Verification items for the finished model (mm, model axes). Face numbers are marked on the shaded views. A direction names the side the tool comes from. Coordinates: 2 decimals unless noted, no trailing zeros. Order: outer loops, then holes, each group sorted by start corner. A loop starts at its lowest first (then second) coordinate and runs counter-clockwise, first axis right, second up. Notation, with made-up numbers: M 82,61.5 L 112,61.5 A17 cw 112,81.5 Z; hole C 85.5,-39 d6. An arc over 180 degrees is marked long. Use one line per item in the form item = value. Start each with the question number.
```python
from build123d import *

# Parameters (mm, degrees)
SKETCH1_W           = 3.5
SKETCH1_H           = 4
SKETCH2_R           = 2
BOSS_EXTRUDE1_DEPTH = 20
SKETCH3_R           = 2
BOSS_EXTRUDE2_DEPTH = 20
CUT_EXTRUDE1_DEPTH  = 2.4


with BuildPart() as part:
    # Sketch1 → Revolve1 (revolve)
    with BuildSketch(Plane.XZ, mode=Mode.PRIVATE) as revolve1_sk:
        with Locations((1.75, 2)):
            Rectangle(SKETCH1_W, SKETCH1_H)
    revolve(revolve1_sk.sketch.rotate(Axis((0, 0, 4), (0, 0, -1)), 180), axis=Axis((0, 0, 4), (0, 0, -1)))

    # Sketch2 → Boss-Extrude1 (add)
    with BuildSketch(Plane.XY.offset(4)):
        Circle(SKETCH2_R)
    extrude(amount=BOSS_EXTRUDE1_DEPTH)

    # Sketch3 → Boss-Extrude2 (add)
    with BuildSketch(Plane.XY.offset(24)):
        Circle(SKETCH3_R)
    extrude(amount=BOSS_EXTRUDE2_DEPTH)

    # Sketch4 → Cut-Extrude1 (cut)
    with BuildSketch(Plane(origin=(0, 0, 0), x_dir=(-1, 0, 0), z_dir=(0, 0, -1))):
        Polygon((-1.7, 0), (-0.85, -1.472243186), (0.85, -1.472243186), (1.7, 0), (0.85, 1.472243186), (-0.85, 1.472243186), align=None)
    extrude(amount=-CUT_EXTRUDE1_DEPTH, mode=Mode.SUBTRACT)


solid = part.part
```
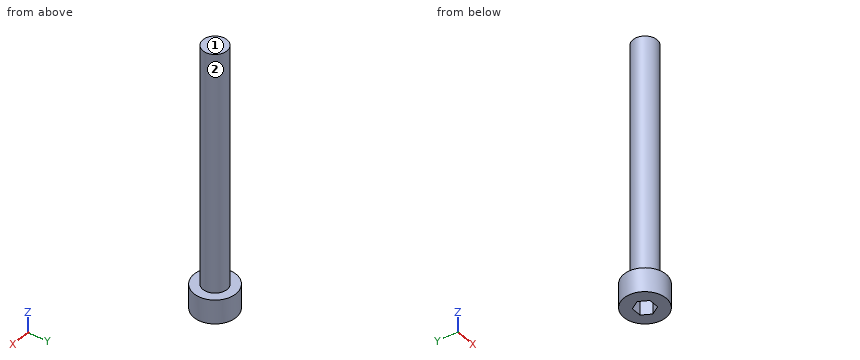
1. Cross-section at B-B on y = -0.75. Enter the section's corners in (x, z), and give its area (3 significant figures).
2. Material ranges on line 1 along Y through (x, z) = (0, 41); line 2 along Z through (x, y) = (-2.25, -2.25); line 3 along Y through (x, z) = (-1.5, 26), recorded low to high.
3. Cross-section at C-C on z = 39. Enter the section's corners in (x, y).
4. Tool access check on the marked faces 1 and 2. Record the directions out of +Z, -Z, +X, -X, +Y, -Y that give a thin tool (end or side, any length) a straight path to the whole face; none if there is none.
5. Depth check by flat-ended pin: P1, Ø2, axis at x = 2.5, z = 27.5, coming from the -Y side; P2, Ø2, axis at y = 0.5, z = 26.5, coming from the +X side; P3, Ø3, axis at y = 2.5, z = 9, coming from the +X side. Enter the tip coordinate at first touch or a pass-through.
6. Cross-section at D-D on y = -2.5. Enter the section's corners in (x, z), and give its area (3 significant figures).
7. Cross-section at A-A on x = 0. Enter the section's corners in (y, z).
Final values:
q1.outline = M -3.42,0 L -1.27,0 L -1.27,2.4 L 1.27,2.4 L 1.27,0 L 3.42,0 L 3.42,4 L 1.85,4 L 1.85,44 L -1.85,44 L -1.85,4 L -3.42,4 Z
q1.area = 170 mm2
q2.line_1 = -2 to 2
q2.line_2 = 0 to 4
q2.line_3 = -1.32 to 1.32
q3.outline = C 0,0 d4
q4.face_1 = +Z, +X, -X, +Y, -Y
q4.face_2 = +Z
q5.P1 = -1.32
q5.P2 = 2
q5.P3 = 1.73
q6.outline = M -2.45,0 L 2.45,0 L 2.45,4 L -2.45,4 Z
q6.area = 19.6 mm2
q7.outline = M -3.5,0 L -1.47,0 L -1.47,2.4 L 1.47,2.4 L 1.47,0 L 3.5,0 L 3.5,4 L 2,4 L 2,44 L -2,44 L -2,4 L -3.5,4 Z
